The listing builds one solid part. Answer for the finished solid, in the listing's coordinates (mm). A direction names the side the tool comes from. Round coordinates to 2 decimals unless told otherwise and drop trailing zeros. Order: outer loops, then holes, each group sorted by start corner. A loop starts at its lowest first (then second) coordinate and runs counter-clockwise, first axis right, second up. Notation, with made-up numbers: (16.5, 49.5) - (34.5, 49.5) arc R30 cw to (34.5, 73.5) - close; hole circle Ø9 at (3, -11). An arc over 180 degrees is marked (long way). One line per item, written item: value. Start each with the question number.
1. A tool of negligible diameter and unlimited length cuts with its end or side. For faces 4 (the cylindrical face through (3.233, 1.341, 1.482)), 5 (the cylindrical face through (-0.58, -1.02, 1.33)), from which of +Z, -Z, +X, -X, +Y, -Y can it reach the whole face along a straight path? Write none if from no direction.
2. Section B-B, the plane z = 7 is taken. Give the vertices of the cut face in (x, y), then the cut area to 3 significant figures.
3. Section A-A, the plane y = 0 is taken. Give the vertices of the cut face in (x, z), then the cut area to 3 significant figures.
4. Flat-ended cylindrical pins translate along their axes: P1, Ø1, axis at x = 0, z = 10.5, coming from the -Y side; P2, Ø1, axis at x = 0, y = 0, coming from the -Z side; P3, Ø1.5, axis at x = -2, y = 2.5, coming from the +Z side. Find the tip coordinate at first contact, or state that the pin passes through.
5. Straight lines are drawn through the part: line 1 (Z direction, x = -2, y = 1.5); line 2 (X direction, y = -1, z = 6.25); line 3 (Z direction, x = -0.25, y = 0). For each, find the intervals that lie inside material, in ascending order.
6. For a pull along X with two mould halves and no side action, classify faces 1 (the cylindrical face through (0, 2, 13)), 2 (the flat face through (-0.8, 1.5, 0)), 3 (the cylindrical face through (0.673, -1.142, 0.071)) as released by +X, released by -X, zero draft, split by the parting line, or undercut.
Autodesk Inventor part; units mm, degrees
ref_plane "YZ Plane" through (0, 0, 0) normal (1, 0, 0) x (0, 1, 0)
ref_plane "XZ Plane" through (0, 0, 0) normal (0, 1, 0) x (-1, 0, 0)
ref_plane "XY Plane" through (0, 0, 0) normal (0, 0, 1) x (1, 0, 0)
sketch "Esquisse1" plane through (0, 0, 0) normal (0, 0, 1) x (1, 0, 0)
  circle A0 centre (0, 0) radius 3.5
  dimension "d0" = 7
extrude "Extrusion1" add sketch "Esquisse1" along normal blind 3
sketch "Esquisse2" plane through (0, 0, 3) normal (0, 0, 1) x (1, 0, 0)
  circle A0 centre (0, 0) radius 3.5
  circle A1 centre (0, 0) radius 2
  dimension "d3" = 4
extrude "Extrusion2" add sketch "Esquisse2" along normal blind 20 contours A1
fillet "Congé1" radius 0.5 1 edges at (-2, 0, 23)
thread "Filetage1"
fillet "Congé2" radius 0.25 2 edges at (-3.5, 0, 0) (-3.5, 0, 3)
sketch "Esquisse3" plane through (0, 0, 0) normal (0, 0, -1) x (-1, 0, 0)
  circle A0 centre (0, 0) radius 3.25
  line L0 (0, 1.4434) -> (1.25, 0.7217)
  line L1 (1.25, 0.7217) -> (1.25, -0.7217)
  line L2 (1.25, -0.7217) -> (0, -1.4434)
  line L3 (0, -1.4434) -> (-1.25, -0.7217)
  line L4 (-1.25, -0.7217) -> (-1.25, 0.7217)
  line L5 (-1.25, 0.7217) -> (0, 1.4434)
  dimension "d10" = 2.5
extrude "Extrusion3" cut sketch "Esquisse3" against normal blind 1.4 contours L0 L1 L2 L3 L4 L5
fillet "Congé3" radius 0.25 12 edges at (-0.625, 1.0825, 0) (-1.25, 0, 0) (-0.625, -1.0825, 0) (0.625, -1.0825, 0) (1.25, 0, 0) (0.625, 1.0825, 0) (-0.625, 1.0825, 1.4) (0.625, 1.0825, 1.4) (1.25, 0, 1.4) (0.625, -1.0825, 1.4) (-0.625, -1.0825, 1.4) (-1.25, 0, 1.4)
fillet "Congé4" radius 0.25 1 edges at (-2, 0, 3)
properties part number "Vis-Pivot" material "Acier"
Answer list:
1. face 4: +Z, -Z
1. face 5: -Z
2. outline: circle Ø4 at (0, 0)
2. area: 12.6 mm²
3. outline: (-3.5, 0.25) arc R0.25 ccw to (-3.25, 0) - (-1.5, 0) arc R0.25 ccw to (-1.25, 0.25) - (-1.25, 1.15) arc R0.25 cw to (-1, 1.4) - (1, 1.4) arc R0.25 cw to (1.25, 1.15) - (1.25, 0.25) arc R0.25 ccw to (1.5, 0) - (3.25, 0) arc R0.25 ccw to (3.5, 0.25) - (3.5, 2.75) arc R0.25 ccw to (3.25, 3) - (2.25, 3) arc R0.25 cw to (2, 3.25) - (2, 22.5) arc R0.5 ccw to (1.5, 23) - (-1.5, 23) arc R0.5 ccw to (-2, 22.5) - (-2, 3.25) arc R0.25 cw to (-2.25, 3) - (-3.25, 3) arc R0.25 ccw to (-3.5, 2.75) - close
3. area: 97.4 mm²
4. P1: stops at y = -2
4. P2: stops at z = 1.4
4. P3: stops at z = 3
5. line 1: z = 0 to 3
5. line 2: x = -1.73 to 1.73
5. line 3: z = 1.4 to 23
6. face 1: split by the parting line
6. face 2: zero draft
6. face 3: undercut
